Verification items for this drawing (mm, ordinates from the low corner). A direction names the side the tool comes from. Coordinates: 2 decimals unless noted, no trailing zeros. Write each loop counter-clockwise with the first axis right and the second up, starting at its lowest first coordinate (ties: lowest second). Pieces come first, ordered by that corner, then holes. Notation, with made-up numbers: (64, -35.75) -> (69, -35.75) arc R29 cw to (69, -8.75) -> close; hole circle Ø10 at (-9, -37.75). An arc over 180 degrees is marked (long way). Answer as CSV lines item,"result".
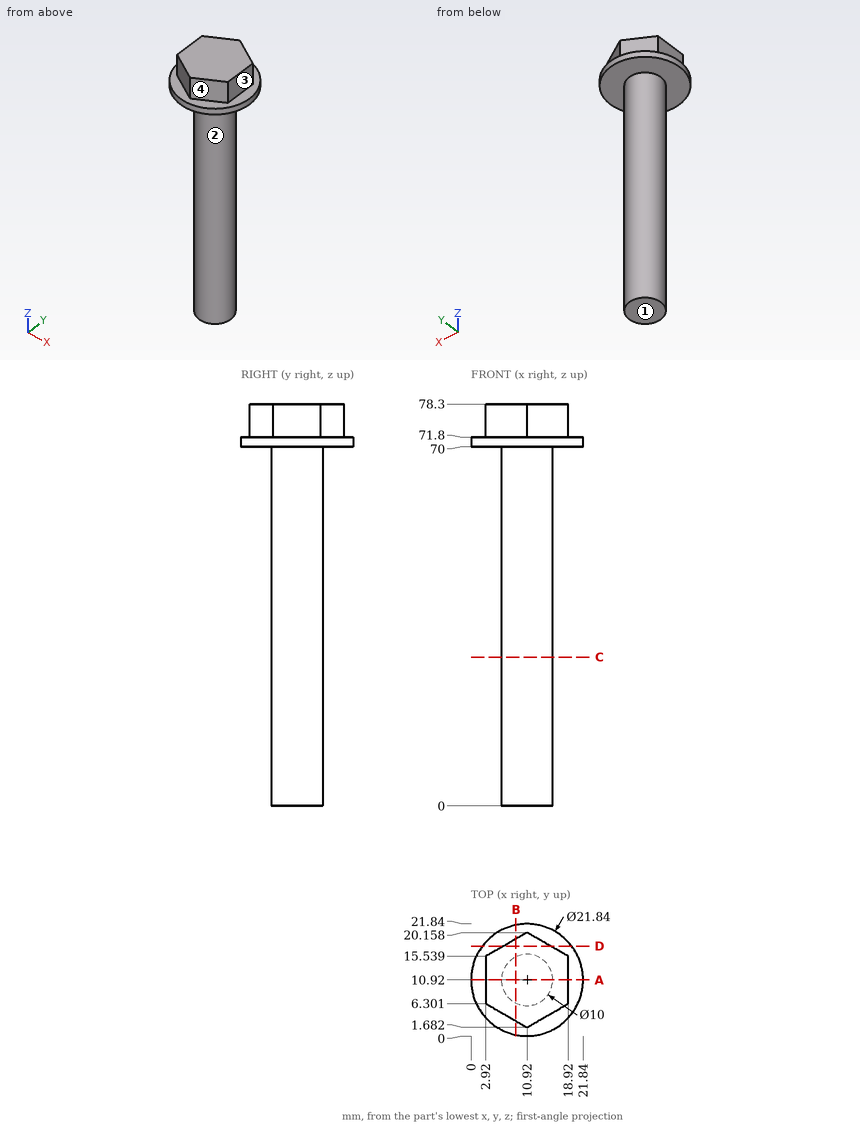
Item 1: Thickness scan on probe 1 along Z at (x, y) = (12.25, 16.5); probe 2 along Z at (x, y) = (2.5, 6.5); probe 3 along Y at (x, z) = (7, 37) (1 decimal). Record the ranges inside material, lowest first.
Responses:
probe 1,"z = 70 to 78.3"
probe 2,"z = 70 to 71.8"
probe 3,"y = 7.8 to 14"
Item 2: Cross-section at C-C, the plane z = 29. Record the cut outline in (x, y).
Responses:
outline,"circle Ø10 at (10.92, 10.92)"
Item 3: Set-up check for the marked faces 1, 2, 3 and 4: record each of +Z, -Z, +X, -X, +Y, -Y from which the full face is reachable in a straight line by a thin tool's end or side.
Responses:
face 1,"-Z, +X, -X, +Y, -Y"
face 2,"-Z"
face 3,"+Z, +X, +Y, -Y"
face 4,"+Z, +X, -Y"
Item 4: Depth check by flat-ended pin: pin 1 Ø1.5 at (x, y) = (2.5, 8) entering from -Z; pin 2 Ø8 at (x, z) = (11.5, 30.5) entering from +Y; pin 3 Ø3 at (y, z) = (12.5, 56.5) entering from +X; pin 4 Ø6.5 at (x, y) = (16, 14.5) entering from -Z. Enter the tip coordinate at first touch or a pass-through.
Responses:
pin 1,"stops at z = 70"
pin 2,"stops at y = 15.92"
pin 3,"stops at x = 15.92"
pin 4,"stops at z = 0"
Item 5: Cross-section at B-B, the plane x = 8.75. Record the cut outline in (y, z) (1 decimal), plus the area to 3 significant figures.
Responses:
outline,"(0.2, 70) -> (6.4, 70) -> (6.4, 0) -> (15.4, 0) -> (15.4, 70) -> (21.6, 70) -> (21.6, 71.8) -> (18.9, 71.8) -> (18.9, 78.3) -> (2.9, 78.3) -> (2.9, 71.8) -> (0.2, 71.8) -> close"
area,"773 mm2"
Item 6: Cross-section at D-D, the plane y = 17.5. Record the cut outline in (x, z) (1 decimal).
Responses:
outline,"(2.2, 70) -> (19.6, 70) -> (19.6, 71.8) -> (15.5, 71.8) -> (15.5, 78.3) -> (6.3, 78.3) -> (6.3, 71.8) -> (2.2, 71.8) -> close"
Item 7: Cross-section at A-A, the plane y = 10.92. Record the cut outline in (x, z).
Responses:
outline,"(0, 70) -> (5.92, 70) -> (5.92, 0) -> (15.92, 0) -> (15.92, 70) -> (21.84, 70) -> (21.84, 71.8) -> (18.92, 71.8) -> (18.92, 78.3) -> (2.92, 78.3) -> (2.92, 71.8) -> (0, 71.8) -> close"
